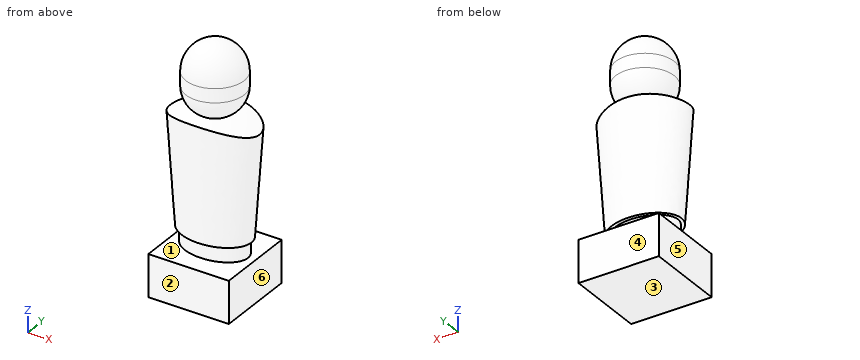
```python
from build123d import *

# Parameters (mm, degrees)
F0_W     = 14.605
F0_H     = 14.605
F1_DEPTH = 7.62
F3_DEPTH = 2.921


with BuildPart() as f1:
    # F0 (on Top) → F1 (new body)
    with BuildSketch(Plane.XY):
        Rectangle(F0_W, F0_H)
    extrude(amount=F1_DEPTH)

    # F2 (on face) → F3 (join)
    with BuildSketch(Plane.XY.offset(7.62)):
        with BuildLine():
            add(Edge.make_bspline(
                [(-5.9944, 0), (-5.9944, -6.8190840294), (2.9972, -3.4095420147), (11.9888, 0), (2.9972, 3.4095420147), (-5.9944, 6.8190840294), (-5.9944, 0)],
                knots=[0, 0, 0, 2.0943951024, 2.0943951024, 4.1887902048, 4.1887902048, 6.2831853072, 6.2831853072, 6.2831853072], degree=2, weights=[1, 0.5, 1, 0.5, 1, 0.5, 1]))
        make_face()
    extrude(amount=F3_DEPTH)

    # F5 (on face) → F7 section 0
    with BuildSketch(Plane.XY.offset(10.541)):
        with BuildLine():
            add(Edge.make_bspline(
                [(6.6294, 0), (6.6294, 7.9189362922), (-3.3147, 3.9594681461), (-13.2588, 0), (-3.3147, -3.9594681461), (6.6294, -7.9189362922), (6.6294, 0)],
                knots=[0, 0, 0, 2.0943951024, 2.0943951024, 4.1887902048, 4.1887902048, 6.2831853072, 6.2831853072, 6.2831853072], degree=2, weights=[1, 0.5, 1, 0.5, 1, 0.5, 1]))
        make_face()
    # F6 (on offset) → F7 section 1
    with BuildSketch(Plane.XY.offset(31.877)):
        with BuildLine():
            add(Edge.make_bspline(
                [(8.255, 0), (8.255, 9.018788555), (-4.1275, 4.5093942775), (-16.51, 0), (-4.1275, -4.5093942775), (8.255, -9.018788555), (8.255, 0)],
                knots=[0, 0, 0, 2.0943951024, 2.0943951024, 4.1887902048, 4.1887902048, 6.2831853072, 6.2831853072, 6.2831853072], degree=2, weights=[1, 0.5, 1, 0.5, 1, 0.5, 1]))
        make_face()
    loft()

    # F8 (on Front) → F9 (revolve, intersect)
    with BuildSketch(Plane.XZ):
        with BuildLine():
            Line((7.3025, 0), (15.24, 24.422544986))
            ThreePointArc((15.24, 24.422544986), (0, 31.8560935557), (-15.24, 24.422544986))
            Line((-15.24, 24.422544986), (-7.3025, 0))
            Line((-7.3025, 0), (7.3025, 0))
        make_face()
    revolve(axis=Axis((0, 0, 0), (-1, 0, 0)), mode=Mode.INTERSECT)

    # F10 (on Front) → F11 (revolve)
    with BuildSketch(Plane.XZ):
        with BuildLine():
            ThreePointArc((-5.2916666667, 36.1427071672), (-3.7126915786, 32.5537193001), (0, 31.2928))
            Line((0, 31.2928), (0, 43.9928))
            ThreePointArc((0, 43.9928), (-3.7440562275, 42.4184357163), (-5.2916666667, 38.6632417318))
            Line((-5.2916666667, 38.6632417318), (-5.2916666667, 36.1427071672))
        make_face()
    revolve(axis=Axis((0, 0, 37.6428), (0, 0, 1)))


solid = f1.part
```
Read the model definition and answer for the solid it produces. Units are mm, in the model's axes. Face numbers are marked on the shaded views. A direction names the side the tool comes from. Coordinates: 2 decimals unless noted, no trailing zeros. Loops run counter-clockwise (first coordinate to the right, second up) from the corner with the lowest first, then second, coordinate; pieces in that order, holes last.
(1) The part is cut by section B-B (z = 37.5). Determine the outline of the cut face in (x, y), and give its area (3 significant figures).
Solution:
outline: circle Ø10.58 at (0, 0)
area: 88.0 mm2
(2) The mould has two halves that part along Z. Classify the marked faces 1, 2 and 3: released by +Z, released by -Z, zero draft, split by the parting line, or undercut.
Solution:
face 1: undercut
face 2: zero draft
face 3: released by -Z
(3) A tool of negligible diameter and unlimited length cuts with its end or side. For the marked faces 4, 5 and 6, from which of +Z, -Z, +X, -X, +Y, -Y can it reach the whole face along a straight path? Write none if from no direction.
Solution:
face 4: +Z, -Z, +X, -X, +Y
face 5: -Z, -X, +Y, -Y
face 6: -Z, +X, +Y, -Y
(4) Consider line 1 along X through (y, z) = (2, 5); line 2 along Z through (x, y) = (6.5, 5.5); line 3 along Z through (x, y) = (1.75, -3.5). Determine where each line is inside the solid, lowest interval first.
Solution:
line 1: x = -7.3 to 7.3
line 2: z = 0 to 7.62
line 3: z = 0 to 31.58, 32.75 to 42.24
(5) Flat-ended cylindrical pins translate along their axes: pin 1 Ø8.5 at (y, z) = (-3, 2) entering from +X; pin 2 Ø2 at (y, z) = (1, 30.5) entering from -X; pin 3 Ø4 at (x, z) = (3, 21) entering from -Y. Find the tip coordinate at first contact, or state that the pin passes through.
Solution:
pin 1: stops at x = 7.3
pin 2: stops at x = -8.12
pin 3: stops at y = -4.85
(6) The part is cut by section A-A (y = -6). Determine the outline of the cut face in (x, z), and give its area (3 significant figures).
Solution:
outline: (-7.3, 0) - (7.3, 0) - (7.3, 7.62) - (-7.3, 7.62) - close
area: 111 mm2
